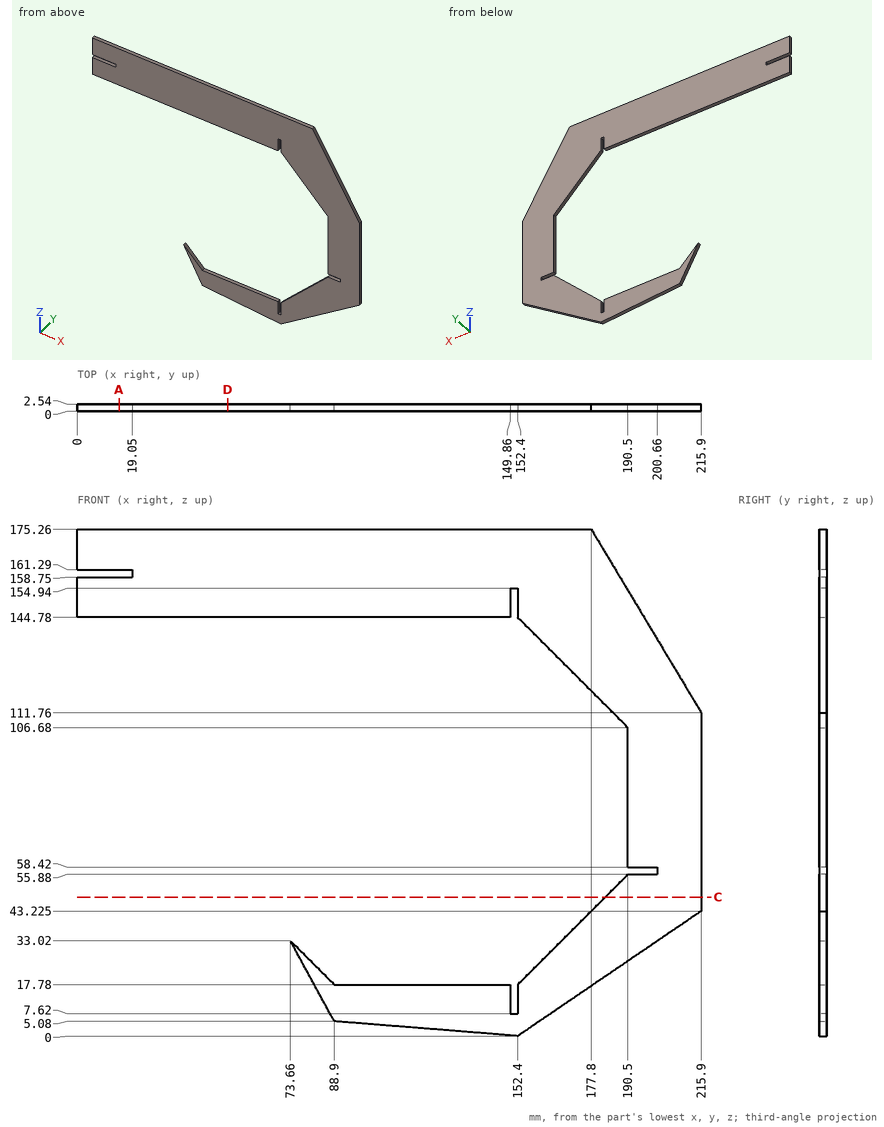
Geometry check sheet. Reference: drawing and pictorial views, mm from the part's lowest x, y, z. Coordinates: 2 decimals unless noted, no trailing zeros. Write each loop counter-clockwise with the first axis right and the second up, starting at its lowest first coordinate (ties: lowest second). Pieces come first, ordered by that corner, then holes. Notation, with made-up numbers: M -39,65.25 L -31,65.25 A16 ccw -31,90.25 Z; hole C 80,35 d6. An arc over 180 degrees is marked long. Write item = value, one per line. Start each with the question number.
1. Thickness scan on probe 1 along Z at (x, y) = (13.5, 0.8); probe 2 along X at (y, z) = (2.45, 102.5); probe 3 along Z at (x, y) = (129, 2.05). Record the ranges inside material, lowest first.
2. Sectioned sample at D-D (x = 52). Record the cut outline in (y, z).
3. Sectioned sample at C-C (z = 48). Record the cut outline in (x, y).
4. Go/stop test with flat-tipped pins: pin 1 (0.8 mm diameter, centred on y = 2, z = 11, fed in from -X); pin 2 (1.3 mm diameter, centred on y = 1.5, z = 57.5, fed in from -X); pin 3 (0.8 mm diameter, centred on y = 1, z = 14, fed in from +X) (1 decimal). Record where each tip stops, or that it passes through.
5. Sectioned sample at A-A (x = 14.5). Record the cut outline in (y, z).
The answers:
q1.probe_1 = 144.78 to 158.75, 161.29 to 175.26
q1.probe_2 = 190.5 to 215.9
q1.probe_3 = 1.87 to 17.78, 144.78 to 175.26
q2.outline = M 0,144.78 L 2.54,144.78 L 2.54,175.26 L 0,175.26 Z
q3.outline = M 182.62,0 L 215.9,0 L 215.9,2.54 L 182.62,2.54 Z
q4.pin_1 = 85.45
q4.pin_2 = 200.66
q4.pin_3 = 173.6
q5.outline = M 0,144.78 L 2.54,144.78 L 2.54,158.75 L 0,158.75 Z; M 0,161.29 L 2.54,161.29 L 2.54,175.26 L 0,175.26 Z
